Autodesk Inventor part; units mm, degrees
ref_plane "YZ Plane" through (0, 0, 0) normal (1, 0, 0) x (0, 1, 0)
ref_plane "XZ Plane" through (0, 0, 0) normal (0, 1, 0) x (-1, 0, 0)
ref_plane "XY Plane" through (0, 0, 0) normal (0, 0, 1) x (1, 0, 0)
sketch "スケッチ1" plane through (0, 0, 0) normal (0, 0, 1) x (1, 0, 0)
  arc A0 (-16.2703, -9.5731) -> (-13.6889, -8.0827) centre (-16.2703, -6.5923) ccw
  arc A1 (-16.2703, -9.5731) -> (-17.2313, -10.1279) centre (-16.2703, -10.6827) ccw
  arc A2 (-17.2313, -10.1279) -> (-17.2313, -11.2375) centre (-16.2703, -10.6827) ccw
  arc A3 (-17.2313, -14.2183) -> (-17.2313, -11.2375) centre (-19.8127, -12.7279) ccw
  arc A4 (-17.2313, -14.2183) -> (-17.2313, -15.3279) centre (-16.2703, -14.7731) ccw
  arc A5 (-17.2313, -15.3279) -> (-16.2703, -15.8827) centre (-16.2703, -14.7731) ccw
  arc A6 (-13.6889, -17.3731) -> (-16.2703, -15.8827) centre (-16.2703, -18.8635) ccw
  arc A7 (-13.6889, -17.3731) -> (-12.7279, -17.9279) centre (-12.7279, -16.8183) ccw
  arc A8 (-12.7279, -17.9279) -> (-11.767, -17.3731) centre (-12.7279, -16.8183) ccw
  arc A9 (-9.1855, -15.8827) -> (-11.767, -17.3731) centre (-9.1855, -18.8635) ccw
  arc A10 (-9.1855, -15.8827) -> (-8.2246, -15.3279) centre (-9.1855, -14.7731) ccw
  arc A11 (-8.2246, -15.3279) -> (-8.2246, -14.2183) centre (-9.1855, -14.7731) ccw
  arc A12 (-8.2246, -11.2375) -> (-8.2246, -14.2183) centre (-5.6431, -12.7279) ccw
  arc A13 (-8.2246, -11.2375) -> (-8.2246, -10.1279) centre (-9.1855, -10.6827) ccw
  arc A14 (-8.2246, -10.1279) -> (-9.1855, -9.5731) centre (-9.1855, -10.6827) ccw
  arc A15 (-11.767, -8.0827) -> (-9.1855, -9.5731) centre (-9.1855, -6.5923) ccw
  arc A16 (-11.767, -8.0827) -> (-12.7279, -7.5279) centre (-12.7279, -8.6375) ccw
  arc A17 (-12.7279, -7.5279) -> (-13.6889, -8.0827) centre (-12.7279, -8.6375) ccw
  circle A18 centre (-12.7279, -12.7279) radius 1.5 construction
  circle A19 centre (-12.7279, -12.7279) radius 1.5
  circle A20 centre (-12.7279, -12.7279) radius 6
  point P0 (0, 0)
  point P1 (0, 0)
  dimension "d0" = 3
extrude "押し出し1" add sketch "スケッチ1" against normal blind 1.5 contours A0 A17 A16 A15 A14 A13 A12 A11 A10 A9 A8 A7 A6 A5 A4 A3 A2 A1 | A20
extrude "押し出し2" add sketch "スケッチ1" along normal blind 4.5 contours A0 A17 A16 A15 A14 A13 A12 A11 A10 A9 A8 A7 A6 A5 A4 A3 A2 A1
chamfer "面取り1" distance 2.7 angle 45 1 edges at (-14.2279, -12.7279, -1.5)
properties part number "原動節接続部v2内-1" material "アルミニウム 2014-T4"
Build history of the part. All positions in model axes, mm. A direction names the side the tool comes from. Round coordinates to 2 decimals unless told otherwise and drop trailing zeros. Write each loop counter-clockwise with the first axis right and the second up, starting at its lowest first coordinate (ties: lowest second). Pieces come first, ordered by that corner, then holes. Notation, with made-up numbers: M 15.5,77.5 L 63.5,77.5 A12 cw 63.5,91.5 Z; hole C 62.5,-16.5 d5. An arc over 180 degrees is marked long. Answer as a JSON object with one key per item and string values. Group by question number.
(1) Flat gauge pin, fed straight in: pin 1 (3 mm diameter, centred on y = -8, z = 0, fed in from -X). Where does the tip first touch, or does it go through?
(2) Drill centre lines: L1, parallel to X at y = -11.75, z = 3.9; L2, parallel to Z at x = -14.75, y = -17; L3, parallel to Y at x = -13.75, z = 3. Where is each one in solid material? Low to high.
(3) Cut at B-B (z = -0.95). Give the cut face in (x, y), and give its area (3 significant figures).
(4) Which spindle directions (+Z, -Z, +X, -X, +Y, -Y) get a long thin tool onto all of the face, cutting with end or side? Do faces 4 (the cylindrical face through (-17.38, -14.78, 2.22)), 5 (the cylindrical face through (-12.18, -7.673, 2.218)), 6 (the cylindrical face through (-10.69, -16.29, 2.22)), 7 (the cylindrical face through (-8.624, -12.75, 2.218)), 8 (the cylindrical face through (-13.29, -7.68, 2.22)). Say none if no direction does.
(5) Cut at A-A (z = 3.75). Give the cut face in (x, y).
(6) Mould opens along Y. For faces 1 (the cylindrical face through (-14.8, -16.27, 2.22)), 2 (the cylindrical face through (-10.657, -9.185, 2.218)), 3 (the cylindrical face through (-8.076, -14.765, 2.218)) say: pulls with the +Y half, pulls with the -Y half, needs draft (parallel to the pull), parting line crosses it, or undercut.
Responses:
{
 "1": {"pin 1": "stops at x = -17.79"},
 "2": {"L1": "x = -17 to -13.87, -11.59 to -8.46", "L2": "z = -1.5 to 0", "L3": "y = -17.27 to -13.83, -11.63 to -8.18"},
 "3": {"outline": "C -12.73,-12.73 d12; hole C -12.73,-12.73 d7.3", "area": "71.2 mm2"},
 "4": {"face 4": "+Z, -X", "face 5": "+Z, +X, +Y", "face 6": "+Z, +X, -Y", "face 7": "+Z, +X", "face 8": "+Z, -X, +Y"},
 "5": {"outline": "M -17.23,-15.33 A1.11 ccw -16.27,-15.88 A2.98 cw -13.69,-17.37 A1.11 ccw -12.73,-17.93 A1.11 ccw -11.77,-17.37 A2.98 cw -9.19,-15.88 A1.11 ccw -8.22,-15.33 A1.11 ccw -8.22,-14.22 A2.98 cw -8.22,-11.24 A1.11 ccw -8.22,-10.13 A1.11 ccw -9.19,-9.57 A2.98 cw -11.77,-8.08 A1.11 ccw -12.73,-7.53 A1.11 ccw -13.69,-8.08 A2.98 cw -16.27,-9.57 A1.11 ccw -17.23,-10.13 A1.11 ccw -17.23,-11.24 A2.98 cw -17.23,-14.22 A1.11 ccw Z; hole C -12.73,-12.73 d3"},
 "6": {"face 1": "pulls with the -Y half", "face 2": "pulls with the +Y half", "face 3": "undercut"}
}
